Read the model definition and answer for the solid it produces. Units are mm, in the model's axes. A direction names the side the tool comes from. Coordinates: 2 decimals unless noted, no trailing zeros. Write each loop counter-clockwise with the first axis right and the second up, starting at its lowest first coordinate (ties: lowest second). Pieces come first, ordered by that corner, then holes.
Item 1: Section D-D (x = 21.5) is taken. Give the vertices of the cut face in (y, z), then the cut area to 3 significant figures.
Item 2: Section A-A (x = -29.5) is taken. Give the vertices of the cut face in (y, z), then the cut area to 3 significant figures.
Item 3: A tool of negligible diameter and unlimited length cuts with its end or side. For faces 1 (the face through (22, 3, -37.397)), 2 (the face through (-26.917, 3.131, -41.172)), 3 (the face through (2.386, 3.219, -34.643)), from which of +Z, -Z, +X, -X, +Y, -Y can it reach the whole face along a straight path? Write none if from no direction.
Item 4: Section B-B (y = 3.25) is taken. State how many separate pieces and enclosed holes the cut face has, then the cut area to 3 significant figures.
Item 5: Determine the mould class of faces 4 (the face through (62.189, 3.219, -15.598)), 5 (the face through (-88.783, 3.131, 22.2)), 6 (the face through (38.03, 3.22, -36.95)) for opening direction Z: released by +Z, released by -Z, zero draft, split by the parting line, or undercut.
Item 6: Section C-C (x = 57.15) is taken. Give the vertices of the cut face in (y, z), then the cut area to 3 significant figures.
Item 7: Straight lines are drawn through the part: probe 1 along X at (y, z) = (0.5, -33); probe 2 along X at (y, z) = (0.5, -20); probe 3 along X at (y, z) = (2.75, -4). For each, find the intervals that lie inside material, in ascending order.
Item 8: Each of these flat-tipped pins is pushed along its axis until it touches: P1, Ø2, axis at y = 3.5, z = 29.5, coming from the -X side; P2, Ø1.5, axis at y = 2, z = 20.5, coming from the +X side. Where does it stop, or does it pass through?
Autodesk Fusion 360 part; units mm, degrees
sketch "Sketch1" plane through (0, 0, 0) normal (0, 1, 0) x (1, 0, 0)
  line L0 (-101.6, 0) -> (-101.6, 19.0663)
  line L1 (-101.6, 19.0663) -> (-69.8663, 50.8)
  line L2 (-69.8663, 50.8) -> (-39.2395, 50.8)
  arc A0 (-33.7037, 26.67) -> (-39.2395, 50.8) centre (-39.2395, 38.1) ccw
  arc A1 (-33.7037, 26.67) -> (-6.7663, 5.5643) centre (-25.4, 9.525) ccw
  line L3 (-6.7663, 5.5643) -> (0, 37.3972)
  line L4 (0, 37.3972) -> (38.1, 37.3972)
  line L5 (38.1, 37.3972) -> (69.85, 19.0663)
  line L6 (69.85, 19.0663) -> (69.85, -19.05)
  line L7 (69.85, -19.05) -> (0, -47.2712)
  line L8 (0, -47.2712) -> (-74.3079, -47.2712)
  line L9 (-74.3079, -47.2712) -> (-101.6, 0)
  dimension "d1" = 9.525
  dimension "d2" = 19.05
  dimension "d3" = 25.4
  dimension "d4" = 102
  dimension "d5" = 38.1
  dimension "d6" = 150
  dimension "d7" = 69.85
  dimension "d8" = 112
  dimension "d9" = 19.05
  dimension "d10" = 120
  dimension "d11" = 101.6
  dimension "d12" = 135
  dimension "d13" = 50.8
  dimension "d14" = 12.7
extrude "Extrude1" add sketch "Sketch1" along normal blind 6.35
fillet "Fillet1" radius 12.7 9 edges at (-69.8663, 3.175, -50.8) (-101.6, 3.175, -19.0663) (-101.6, 3.175, 0) (-74.3079, 3.175, 47.2712) (0, 3.175, 47.2712) (0, 3.175, -37.3972) (38.1, 3.175, -37.3972) (69.85, 3.175, -19.0663) (69.85, 3.175, 19.05)
sketch "Sketch2" plane through (0, 6.35, 0) normal (0, 1, 0) x (-1, 0, 0)
  arc A0 (-61.9075, 22.259) -> (-69.85, 10.4837) centre (-57.15, 10.4837) ccw
  line L0 (-69.85, 10.4837) -> (-69.85, -11.7339)
  arc A1 (-69.85, -11.7339) -> (-63.5, -22.7325) centre (-57.15, -11.7339) ccw
  line L1 (-63.5, -22.7325) -> (-41.047, -35.6957)
  arc A2 (-41.047, -35.6957) -> (-34.697, -37.3972) centre (-34.697, -24.6972) ccw
  line L2 (-34.697, -37.3972) -> (-10.2843, -37.3972)
  arc A3 (-10.2843, -37.3972) -> (2.1382, -27.3376) centre (-10.2843, -24.6972) ccw
  line L3 (2.1382, -27.3376) -> (6.7663, -5.5643)
  arc A4 (33.7037, -26.67) -> (6.7663, -5.5643) centre (25.4, -9.525) ccw
  arc A5 (33.7037, -26.67) -> (39.2395, -50.8) centre (39.2395, -38.1) ccw
  line L4 (39.2395, -50.8) -> (64.6058, -50.8)
  arc A6 (64.6058, -50.8) -> (73.586, -47.0803) centre (64.6058, -38.1) ccw
  line L5 (73.586, -47.0803) -> (97.8803, -22.786)
  arc A7 (97.8803, -22.786) -> (101.6, -13.8058) centre (88.9, -13.8058) ccw
  line L6 (101.6, -13.8058) -> (101.6, -3.403)
  arc A8 (101.6, -3.403) -> (99.8985, 2.947) centre (88.9, -3.403) ccw
  line L7 (99.8985, 2.947) -> (77.9741, 40.9212)
  arc A9 (77.9741, 40.9212) -> (66.9756, 47.2712) centre (66.9756, 34.5712) ccw
  line L8 (66.9756, 47.2712) -> (2.4686, 47.2712)
  arc A10 (2.4686, 47.2712) -> (-2.2889, 46.3465) centre (2.4686, 34.5712) ccw
  line L9 (-2.2889, 46.3465) -> (-61.9075, 22.259)
  circle A11 centre (64.6058, -38.1) radius 6.35
  circle A12 centre (39.2395, -38.1) radius 6.35
  circle A13 centre (-10.2843, -24.6972) radius 6.35
  circle A14 centre (-57.15, -11.7339) radius 6.35
  circle A15 centre (-57.15, 10.4837) radius 6.35
  circle A16 centre (66.9756, 34.5712) radius 6.35
  circle A17 centre (88.9, -3.403) radius 6.35
  dimension "d18" = 12.7
extrude "Extrude2" cut sketch "Sketch2" against normal blind 15.24 contours A11 | A12 | A13 | A14 | A15 | A16 | A17
Established:
1. outline: (0, -37.4) - (6.35, -37.4) - (6.35, 38.58) - (0, 38.58) - close
1. area: 482 mm2
2. outline: (0, -46.25) - (6.35, -46.25) - (6.35, -29.95) - (0, -29.95) - close; (0, 9.08) - (6.35, 9.08) - (6.35, 47.27) - (0, 47.27) - close
2. area: 346 mm2
3. face 1: -Z, +X, +Y, -Y
3. face 2: +Y, -Y
3. face 3: -Z, +Y, -Y
4. separate pieces: 1
4. enclosed holes: 7
4. area: 10,600 mm2
5. face 4: undercut
5. face 5: released by +Z
5. face 6: released by -Z
6. outline: (0, -26.4) - (6.35, -26.4) - (6.35, -18.08) - (0, -18.08) - close; (0, -5.38) - (6.35, -5.38) - (6.35, 4.13) - (0, 4.13) - close; (0, 16.83) - (6.35, 16.83) - (6.35, 24.18) - (0, 24.18) - close
6. area: 160 mm2
7. probe 1: x = -87.67 to -68.39, -60.82 to -43.02, -35.46 to -27.61, 0.67 to 45.72
7. probe 2: x = -99.99 to -41.31, -3.7 to 6.01, 14.56 to 66.79
7. probe 3: x = -101.6 to -95.22, -82.58 to -43.63, -7.17 to 69.85
8. P1: stops at x = -85.15
8. P2: stops at x = 65.83
